from build123d import *

# Parameters (mm, degrees)
RESSALTO_EXTRUS_O3_DEPTH = 5
ESBO_O4_R                = 1.5
CORTE_EXTRUS_O3_DEPTH    = 10


with BuildPart() as part:
    # Esboço1 → Ressalto-extrusão3 (new body)
    with BuildSketch(Plane.XY):
        with BuildLine():
            Line((-31.851570772, -17.801096987), (-27.063885949, -17.801096987))
            Line((-27.063885949, -17.801096987), (10.936114051, -17.801096987))
            Line((10.936114051, -17.801096987), (15.723798874, -17.801096987))
            ThreePointArc((15.723798874, -17.801096987), (21.039894205, -19.331201448), (24.729153299, -23.4532709))
            ThreePointArc((24.729153299, -23.4532709), (27.934250919, -27.635644423), (32.536114051, -30.202306605))
            ThreePointArc((32.536114051, -30.202306605), (35.210937986, -29.759166326), (36.436114051, -27.340489001))
            Line((36.436114051, -27.340489001), (36.436114051, -17.801096987))
            Line((36.436114051, -17.801096987), (36.436114051, 0.198903013))
            add(Edge.make_bspline(
                [(36.436114051, 75.398903013), (24.729153299, 37.798903013), (36.436114051, 0.198903013)],
                knots=[0, 0, 0, 1, 1, 1], degree=2, weights=[1, 3, 1]))
            Line((36.436114051, 75.398903013), (36.436114051, 93.398903013))
            Line((36.436114051, 93.398903013), (36.436114051, 102.938295027))
            ThreePointArc((36.436114051, 102.938295027), (35.210937986, 105.356972352), (32.536114051, 105.800112631))
            ThreePointArc((32.536114051, 105.800112631), (27.934250919, 103.23345045), (24.729153299, 99.051076926))
            ThreePointArc((24.729153299, 99.051076926), (21.039894205, 94.929007474), (15.723798874, 93.398903013))
            Line((15.723798874, 93.398903013), (10.936114051, 93.398903013))
            Line((10.936114051, 93.398903013), (-27.063885949, 93.398903013))
            Line((-27.063885949, 93.398903013), (-31.851570772, 93.398903013))
            ThreePointArc((-31.851570772, 93.398903013), (-37.167666102, 94.929007474), (-40.856925197, 99.051076926))
            ThreePointArc((-40.856925197, 99.051076926), (-44.062022817, 103.23345045), (-48.663885949, 105.800112631))
            ThreePointArc((-48.663885949, 105.800112631), (-51.338709884, 105.356972352), (-52.563885949, 102.938295027))
            Line((-52.563885949, 102.938295027), (-52.563885949, 93.398903013))
            Line((-52.563885949, 93.398903013), (-52.563885949, 75.398903013))
            add(Edge.make_bspline(
                [(-52.563885949, 75.398903013), (-40.856925197, 37.798903013), (-52.563885949, 0.198903013)],
                knots=[0, 0, 0, 1, 1, 1], degree=2, weights=[1, 3, 1]))
            Line((-52.563885949, 0.198903013), (-52.563885949, -17.801096987))
            Line((-52.563885949, -17.801096987), (-52.563885949, -27.340489001))
            ThreePointArc((-52.563885949, -27.340489001), (-51.338709884, -29.759166326), (-48.663885949, -30.202306605))
            ThreePointArc((-48.663885949, -30.202306605), (-44.062022817, -27.635644423), (-40.856925197, -23.4532709))
            ThreePointArc((-40.856925197, -23.4532709), (-37.167666102, -19.331201448), (-31.851570772, -17.801096987))
        make_face()
    extrude(amount=RESSALTO_EXTRUS_O3_DEPTH)

    # Esboço4 → Corte-extrusão3 (cut)
    with BuildSketch(Plane(origin=(0, 0, 0), x_dir=(-1, 0, 0), z_dir=(0, 0, -1))):
        with Locations((-31.436114051, 99.800112631)):
            Circle(ESBO_O4_R)
        with Locations((47.563885949, 99.800112631)):
            Circle(ESBO_O4_R)
        with Locations((8.063885949, 84.898903013)):
            Circle(ESBO_O4_R)
        with Locations((8.063885949, -9.301096987)):
            Circle(ESBO_O4_R)
        with Locations((47.563885949, -24.202306605)):
            Circle(ESBO_O4_R)
        with Locations((-31.436114051, -24.202306605)):
            Circle(ESBO_O4_R)
        with BuildLine():
            Line((-7.436114051, 90.598903013), (-1.436114051, 90.598903013))
            ThreePointArc((-1.436114051, 90.598903013), (-0.021900489, 90.013116575), (0.563885949, 88.598903013))
            Line((0.563885949, 88.598903013), (0.563885949, 78.698903013))
            ThreePointArc((0.563885949, 78.698903013), (-0.021900489, 77.284689451), (-1.436114051, 76.698903013))
            Line((-1.436114051, 76.698903013), (-7.436114051, 76.698903013))
            ThreePointArc((-7.436114051, 76.698903013), (-8.850327613, 77.284689451), (-9.436114051, 78.698903013))
            Line((-9.436114051, 78.698903013), (-9.436114051, 88.598903013))
            ThreePointArc((-9.436114051, 88.598903013), (-8.850327613, 90.013116575), (-7.436114051, 90.598903013))
        make_face()
        with BuildLine():
            Line((17.563885949, 90.598903013), (23.563885949, 90.598903013))
            ThreePointArc((23.563885949, 90.598903013), (24.978099511, 90.013116575), (25.563885949, 88.598903013))
            Line((25.563885949, 88.598903013), (25.563885949, 78.698903013))
            ThreePointArc((25.563885949, 78.698903013), (24.978099511, 77.284689451), (23.563885949, 76.698903013))
            Line((23.563885949, 76.698903013), (17.563885949, 76.698903013))
            ThreePointArc((17.563885949, 76.698903013), (16.149672387, 77.284689451), (15.563885949, 78.698903013))
            Line((15.563885949, 78.698903013), (15.563885949, 88.598903013))
            ThreePointArc((15.563885949, 88.598903013), (16.149672387, 90.013116575), (17.563885949, 90.598903013))
        make_face()
        with BuildLine():
            Line((25.563885949, -13.001096987), (25.563885949, -3.101096987))
            ThreePointArc((25.563885949, -3.101096987), (24.978099511, -1.686883425), (23.563885949, -1.101096987))
            Line((23.563885949, -1.101096987), (17.563885949, -1.101096987))
            ThreePointArc((17.563885949, -1.101096987), (16.149672387, -1.686883425), (15.563885949, -3.101096987))
            Line((15.563885949, -3.101096987), (15.563885949, -13.001096987))
            ThreePointArc((15.563885949, -13.001096987), (16.149672387, -14.415310549), (17.563885949, -15.001096987))
            Line((17.563885949, -15.001096987), (23.563885949, -15.001096987))
            ThreePointArc((23.563885949, -15.001096987), (24.978099511, -14.415310549), (25.563885949, -13.001096987))
        make_face()
        with BuildLine():
            Line((0.563885949, -13.001096987), (0.563885949, -3.101096987))
            ThreePointArc((0.563885949, -3.101096987), (-0.021900489, -1.686883425), (-1.436114051, -1.101096987))
            Line((-1.436114051, -1.101096987), (-7.436114051, -1.101096987))
            ThreePointArc((-7.436114051, -1.101096987), (-8.850327613, -1.686883425), (-9.436114051, -3.101096987))
            Line((-9.436114051, -3.101096987), (-9.436114051, -13.001096987))
            ThreePointArc((-9.436114051, -13.001096987), (-8.850327613, -14.415310549), (-7.436114051, -15.001096987))
            Line((-7.436114051, -15.001096987), (-1.436114051, -15.001096987))
            ThreePointArc((-1.436114051, -15.001096987), (-0.021900489, -14.415310549), (0.563885949, -13.001096987))
        make_face()
    extrude(amount=-CORTE_EXTRUS_O3_DEPTH, mode=Mode.SUBTRACT)


solid = part.part
Build history of the part. All positions in model axes, mm. A direction names the side the tool comes from. Give positions to 0.01 mm unless a question says otherwise; leave off trailing zeros. Loops run counter-clockwise (first coordinate to the right, second up) from the corner with the lowest first, then second, coordinate; pieces in that order, holes last. Notation, with made-up numbers: (65, 24) -> (79, 24) arc R16 cw to (79, 47) -> close; hole circle Ø6 at (-14.75, -8.75). An arc over 180 degrees is marked (long way). Answer in a Markdown table with one row per item.
Item 1: Probe line 1 along Y through (x, z) = (-18, 4.75); line 2 along X through (y, z) = (82.5, 2.25); line 3 along X through (y, z) = (98.5, 1.1). List the from-to ranges inside material, lowest first. Write a range as [from, to].
Findings below:
| item | result |
|---|---|
| line 1 | y = [-17.8, -15], [-1.1, 76.7], [90.6, 93.4] |
| line 2 | x = [-52.56, -25.56], [-15.56, -0.56], [9.44, 36.44] |
| line 3 | x = [-52.56, -48.31], [-46.82, -40.57], [24.44, 30.69], [32.18, 36.44] |
Item 2: Mould opens along X. For faces 1 (the flat face through (-9, 39, 5)), 2 (the flat face through (-15.564, -8, 2)), 3 (the flat face through (36.436, -14, 2)) say: pulls with the +X half, pulls with the -X half, needs draft (parallel to the pull), parting line crosses it, or undercut.
Findings below:
| item | result |
|---|---|
| face 1 | needs draft |
| face 2 | undercut |
| face 3 | pulls with the +X half |
Item 3: Slice it at B-B on x = 21. Write the cut outline in (y, z), plus the area to 3 significant figures.
Findings below:
| item | result |
|---|---|
| outline | (-19.31, 0) -> (94.9, 0) -> (94.9, 5) -> (-19.31, 5) -> close |
| area | 571 mm² |
Item 4: Flat gauge pins, fed straight in: P1, Ø2.5, axis at x = -47.56, y = 99.8, coming from the -Z side; P2, Ø2, axis at x = 22, z = 2.5, coming from the -Y side; P3, Ø2.5, axis at x = 5, z = 2, coming from the +Y side; P4, Ø3, axis at x = -9.5, z = 0.5, coming from the -Y side. Where does each tip first touch, or does it go through?
Findings below:
| item | result |
|---|---|
| P1 | passes through |
| P2 | stops at y = -20.94 |
| P3 | stops at y = 93.4 |
| P4 | stops at y = -17.8 |
Item 5: Tool access for faces 4 (the flat face through (-0.564, -8, 2)), 5 (the flat face through (36.436, 89, 2)), 6 (the flat face through (-8, 93.399, 2)), 7 (the flat face through (-8, -17.801, 2)): list every direction of +Z, -Z, +X, -X, +Y, -Y with a clear straight run to the whole face (end or side of a thin tool).
Findings below:
| item | result |
|---|---|
| face 4 | +Z, -Z |
| face 5 | +Z, -Z, +X, +Y, -Y |
| face 6 | +Z, -Z, +Y |
| face 7 | +Z, -Z, -Y |
Item 6: Slice it at A-A on z = 2.25. Give the number of separate pieces and of enclosed holes in the cut face, plus the area to 3 significant figures.
Findings below:
| item | result |
|---|---|
| separate pieces | 1 |
| enclosed holes | 10 |
| area | 9,080 mm² |
